```python
from build123d import *

# Parameters (mm, degrees)
F3_DEPTH = 50
F4_COUNT = 20


with BuildPart() as f1:
    # F0 (on Top) → F1 (revolve)
    with BuildSketch(Plane.XY):
        Polygon((0, 40), (0, 50), (-50, 50), (-50, 40), (-35, 40), (-35, 32), (-27, 32), (-27, 25.6603773385), (-23, 25.6603773385), (-23, 32), (-15, 32), (-15, 40), align=None)
    revolve(axis=Axis((-25, 0, 0), (-1, 0, 0)))

    # F2 (on face) → F3 (cut)
    with BuildSketch(Plane.YZ):
        with BuildLine():
            Line((1.2014859403, 42.3988246892), (3.9122925633, 49.8467046744))
            ThreePointArc((3.9122925633, 49.8467046744), (0.160266729, 49.9997431451), (-3.5926630814, 49.8707606918))
            Line((-3.5926630814, 49.8707606918), (-0.8731007841, 42.3988246892))
            ThreePointArc((-0.8731007841, 42.3988246892), (-0.5069845997, 41.9216927883), (0.0665918367, 41.7408448326))
            Line((0.0665918367, 41.7408448326), (0.2617933195, 41.7408448326))
            ThreePointArc((0.2617933195, 41.7408448326), (0.8353697558, 41.9216927883), (1.2014859403, 42.3988246892))
        make_face()
    f3 = extrude(amount=-F3_DEPTH, mode=Mode.SUBTRACT)

    # F4: F3 ×20 about axis
    f4_axis = Axis((0, 0, 0), (-1, 0, 0))
    for i in range(1, F4_COUNT):
        add(f3.rotate(f4_axis, i * 360 / F4_COUNT), mode=Mode.SUBTRACT)


solid = f1.part
```
The model under review builds one solid part; all positions refer to its coordinate system, in mm. A direction names the side the tool comes from. Coordinates: 2 decimals unless noted, no trailing zeros. Loops run counter-clockwise (first coordinate to the right, second up) from the corner with the lowest first, then second, coordinate; pieces in that order, holes last. Notation, with made-up numbers: (12, -1.5) -> (23, -1.5) arc R24 cw to (23, 22.5) -> close; hole circle Ø1 at (-4.75, 59.5). An arc over 180 degrees is marked (long way). Answer as CSV lines item,"result".
Item 1: For L1, parallel to Z at x = -40.5, y = 0; L2, parallel to Y at x = -47, z = -42.5, list the stretches that pass through material, from the lowest coordinate up.
Results below:
L1,"z = -41.74 to -40, 40 to 41.74"
L2,"y = -26.34 to -16.24, -12.21 to -1.24, 0.91 to 11.9, 15.84 to 26.1"
Item 2: Machinability: for faces 1 (the flat face through (-24.65, 25.326, 38.69)), 2 (the cylindrical face through (-18.94, -6.94, 31.24)), 3 (the flat face through (-24.65, -2.538, -46.071)), 4 (the flat face through (-24.65, -46.187, -2.252)), 5 (the flat face through (-24.65, 16.65, 43.03)), which of the approach directions +Z, -Z, +X, -X, +Y, -Y give a long, thin tool a straight path to every point of the face, cutting with its end or side? Answer none if there is none.
Results below:
face 1,"+X, -X"
face 2,"+X"
face 3,"-Z, +X, -X"
face 4,"+X, -X, -Y"
face 5,"+Z, +X, -X"
Item 3: Insertion check: pin 1 (10 mm diameter, centred on x = -8.5, z = -22, fed in from +Y); pin 2 (5 mm diameter, centred on y = -7, z = -29.5, fed in from -X); pin 3 (2 mm diameter, centred on x = -41, y = 11, fed in from -Z); pin 4 (19 mm diameter, centred on y = -6.5, z = 9.5, fed in from +X). Each pin has a flat end and moves straight along its axis. Give the tip position at first contact, or say it passes through.
Results below:
pin 1,"stops at y = 46.2"
pin 2,"stops at x = -35"
pin 3,"stops at z = -48.99"
pin 4,"passes through"
Item 4: Draft analysis for pull direction Y (two halves, no side actions). For faces 6 (the cylindrical face through (-25.35, 35.28, -35.43)), 7 (the flat face through (-24.65, 16.414, -43.231)), 8 (the cylindrical face through (-25.4, -44.6, -22.6)), state which applies: +Y half, -Y half, draft (parallel to the pull), parting line (faces both ways), or undercut.
Results below:
face 6,"+Y half"
face 7,"undercut"
face 8,"-Y half"
Item 5: Take a section at B-B, the plane y = 9.5. State the section outline as (x, z) points.
Results below:
outline,"(-50, -49.09) -> (0, -49.09) -> (0, -38.86) -> (-15, -38.86) -> (-15, -30.56) -> (-23, -30.56) -> (-23, -23.84) -> (-27, -23.84) -> (-27, -30.56) -> (-35, -30.56) -> (-35, -38.86) -> (-50, -38.86) -> close; (-50, 38.86) -> (-35, 38.86) -> (-35, 30.56) -> (-27, 30.56) -> (-27, 23.84) -> (-23, 23.84) -> (-23, 30.56) -> (-15, 30.56) -> (-15, 38.86) -> (0, 38.86) -> (0, 49.09) -> (-50, 49.09) -> close"
Item 6: Take a section at A-A, the plane z = 9. State the section outline as (x, y) points.
Results below:
outline,"(-50, -49.18) -> (0, -49.18) -> (0, -38.97) -> (-15, -38.97) -> (-15, -30.71) -> (-23, -30.71) -> (-23, -24.03) -> (-27, -24.03) -> (-27, -30.71) -> (-35, -30.71) -> (-35, -38.97) -> (-50, -38.97) -> close; (-50, 38.97) -> (-35, 38.97) -> (-35, 30.71) -> (-27, 30.71) -> (-27, 24.03) -> (-23, 24.03) -> (-23, 30.71) -> (-15, 30.71) -> (-15, 38.97) -> (0, 38.97) -> (0, 49.18) -> (-50, 49.18) -> close"
